```python
from build123d import *

# Parameters (mm, degrees)
F0_W     = 390
F0_H     = 37
F1_DEPTH = 1.5
F0_H_2   = 70
F0_H_3   = 3
F2_DEPTH = 3


with BuildPart() as f1:
    # F0 (on Top) → F1 (new body)
    with BuildSketch(Plane.XY):
        with Locations((0, 56.5)):
            Rectangle(F0_W, F0_H)
    extrude(amount=F1_DEPTH)



with BuildPart() as f1b:
    # F0 (on Top) → F1, piece 2 (new body)
    with BuildSketch(Plane.XY):
        Rectangle(F0_W, F0_H_2)
    extrude(amount=F1_DEPTH)


with BuildPart() as f1c:
    # F0 (on Top) → F1, piece 3 (new body)
    with BuildSketch(Plane.XY):
        with Locations((0, -56.5)):
            Rectangle(F0_W, F0_H)
    extrude(amount=F1_DEPTH)


with BuildPart() as f1_1:
    add(f1.part)

    add(f1b.part)  # F2 merges F1b

    add(f1c.part)  # F2 merges F1c
    # F0 (on Top) → F2 (join)
    with BuildSketch(Plane.XY):
        with Locations((0, 36.5)):
            Rectangle(F0_W, F0_H_3)
        with Locations((0, -36.5)):
            Rectangle(F0_W, F0_H_3)
    extrude(amount=F2_DEPTH)


solid = f1_1.part
```
Verification items for the finished model (mm, model axes). A direction names the side the tool comes from. Give positions to 0.01 mm unless a question says otherwise; leave off trailing zeros. Order: outer loops, then holes, each group sorted by start corner. A loop starts at its lowest first (then second) coordinate and runs counter-clockwise, first axis right, second up. Notation, with made-up numbers: (82.5, 12.25) - (132.5, 12.25) arc R15 ccw to (132.5, 33.25) - close; hole circle Ø2 at (-27.5, -23). An arc over 180 degrees is marked (long way). Answer as CSV lines item,"result". Start each with the question number.
Item 1: Section check A-A, the plane z = 2.15. Record the boundary of the cut face in (x, y).
Item 2: Access from +Z, -Z, +X, -X, +Y, -Y to the whole of each face (thin tool, end or side, straight path). Record for faces 1 (the face through (-3, 0, 1.5)), 2 (the face through (-3, -56, 1.5)), 3 (the face through (-3, 57, 1.5)), 4 (the face through (-3, 1, 0)).
Item 3: Section check C-C, the plane y = 2.5. Record the boundary of the cut face in (x, z), plus the area to 3 significant figures.
Item 4: Material ranges on L1, parallel to Y at x = -101, z = 2.1; L2, parallel to Z at x = 179.5, y = 47.5, recorded low to high.
Item 5: Gauge pin test, flat ends, axial feed: pin 1 (0.8 mm diameter, centred on x = 63, z = 2, fed in from -Y); pin 2 (1.6 mm diameter, centred on x = -40, z = 2, fed in from +Y); pin 3 (12 mm diameter, centred on x = -107, y = 15, fed in from +Z). Record the tip position at first contact, or that the pin passes through.
Item 6: Section check B-B, the plane x = -61. Record the boundary of the cut face in (y, z), plus the area to 3 significant figures.
Filled in:
1,outline,"(-195, -38) - (195, -38) - (195, -35) - (-195, -35) - close; (-195, 35) - (195, 35) - (195, 38) - (-195, 38) - close"
2,face 1,"+Z, +X, -X"
2,face 2,"+Z, +X, -X, -Y"
2,face 3,"+Z, +X, -X, +Y"
2,face 4,"-Z, +X, -X, +Y, -Y"
3,outline,"(-195, 0) - (195, 0) - (195, 1.5) - (-195, 1.5) - close"
3,area,"585 mm^2"
4,L1,"-38 to -35, 35 to 38"
4,L2,"0 to 1.5"
5,pin 1,"y = -38"
5,pin 2,"y = 75"
5,pin 3,"z = 1.5"
6,outline,"(-75, 0) - (75, 0) - (75, 1.5) - (38, 1.5) - (38, 3) - (35, 3) - (35, 1.5) - (-35, 1.5) - (-35, 3) - (-38, 3) - (-38, 1.5) - (-75, 1.5) - close"
6,area,"234 mm^2"
